Autodesk Fusion 360 part; units mm, degrees
sketch "Sketch1" plane through (0, 0, 0) normal (0, 0, 1) x (1, 0, 0)
  line L0 (0, 0) -> (18.542, 0)
  line L1 (18.542, 0) -> (18.542, 39.37)
  line L2 (18.542, 39.37) -> (0, 39.37)
  line L3 (0, 39.37) -> (0, 0)
  line L4 (3.302, 0) -> (3.302, 39.37)
  line L5 (15.24, 0) -> (15.24, 39.37)
  line L6 (16.51, 38.1) -> (17.272, 38.1)
  line L7 (17.272, 38.1) -> (17.272, 1.27)
  line L8 (17.272, 1.27) -> (16.51, 1.27)
  line L9 (16.51, 1.27) -> (16.51, 38.1)
  line L10 (1.27, 38.1) -> (2.032, 38.1)
  line L11 (2.032, 38.1) -> (2.032, 1.27)
  line L12 (2.032, 1.27) -> (1.27, 1.27)
  line L13 (1.27, 1.27) -> (1.27, 38.1)
  line L14 (-1.6611, 32.385) -> (20.0985, 32.385) construction
  line L15 (-1.6611, 6.985) -> (20.0985, 6.985) construction
  line L16 (8.9225, 41.0496) -> (8.9225, -1.9164) construction
  circle A0 centre (8.9225, 32.385) radius 2.032
  circle A1 centre (8.9225, 6.985) radius 2.032
  dimension "d1" = 18.542
  dimension "d2" = 39.37
  dimension "d3" = 3.302
  dimension "d4" = 3.302
  dimension "d5" = 36.83
  dimension "d6" = 1.27
  dimension "d7" = 0.762
  dimension "d8" = 1.27
  dimension "d9" = 36.83
  dimension "d11" = 0.762
  dimension "d12" = 1.27
  dimension "d13" = 1.27
  dimension "d26" = 6.985
  dimension "d27" = 6.985
  dimension "d28" = 4.064
  dimension "d29" = 4.064
extrude "Extrude1" add sketch "Sketch1" along normal blind 2.54 contours L0 L2 L4 L5 | A0 | A1
extrude "Extrude2" add sketch "Sketch1" along normal blind 12.7 contours L0 L1 L2 L5
extrude "Extrude3" add sketch "Sketch1" along normal blind 12.7 contours L0 L2 L3 L4
extrude "Extrude4" add sketch "Sketch1" along normal blind 6.35 contours L6 L7 L8 L9
extrude "Extrude5" add sketch "Sketch1" along normal blind 6.35 contours L10 L11 L12 L13
extrude "Extrude6" cut sketch "Sketch1" along normal through all contours A0
extrude "Extrude7" cut sketch "Sketch1" along normal through all contours A1
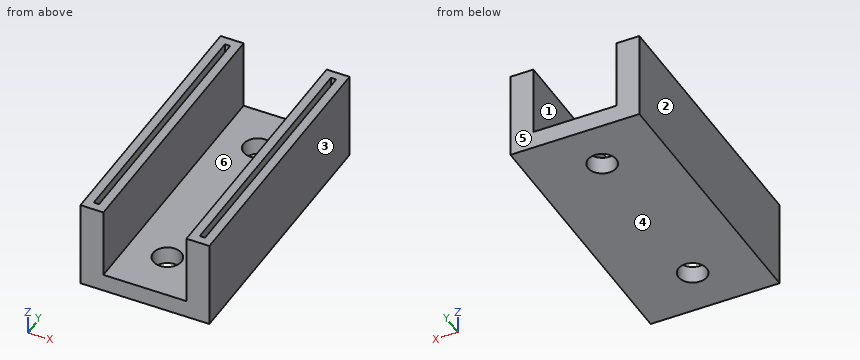
For this review, take the finished solid that the model builds, in its own axes (mm). Face numbers are marked on the shaded views. A direction names the side the tool comes from. Round coordinates to 2 decimals unless told otherwise and drop trailing zeros. Write each loop counter-clockwise with the first axis right and the second up, starting at its lowest first coordinate (ties: lowest second). Pieces come first, ordered by that corner, then holes. Notation, with made-up numbers: M -5.5,31 L 38.5,31 A16 ccw 38.5,43 Z; hole C 52,83.5 d1. An arc over 180 degrees is marked long. One line per item, written item: value. Start each with the question number.
(1) Machinability: for the marked faces 5 and 6, which of the approach directions +Z, -Z, +X, -X, +Y, -Y give a long, thin tool a straight path to every point of the face, cutting with its end or side? Answer none if there is none.
(2) We need section C-C (y = 13). Give the boundary of the cut face in (x, z), and give its area (3 significant figures).
(3) The part is to be moulded in two halves that separate along X. For the marked faces 1, 2, 3 and 4, say which applies: released by +X, released by -X, zero draft, split by the parting line, or undercut.
(4) We need section D-D (y = 34). Give the boundary of the cut face in (x, z).
(5) Wall thickness on line 1 (X direction, y = 17.5, z = 11.5); line 2 (X direction, y = 20.5, z = 4); line 3 (Z direction, x = 10.75, y = 4): over which ranges is each line inside the solid? List them lowest first.
(6) We need section B-B (z = 4). Give the boundary of the cut face in (x, y).
(7) We need section A-A (z = 7.5). Give the boundary of the cut face in (x, y), and give its area (3 significant figures).
(8) Insertion check: pin 1 (3.5 mm diameter, centred on x = 8.92, y = 6.98, fed in from -Z). The pin has a flat end and moves straight along its axis. Give the tip position at first contact, or say it passes through.
Result:
1. face 5: +Z, -Z, +X, -X, +Y
1. face 6: +Z, +Y, -Y
2. outline: M 0,0 L 18.54,0 L 18.54,12.7 L 17.27,12.7 L 17.27,6.35 L 16.51,6.35 L 16.51,12.7 L 15.24,12.7 L 15.24,2.54 L 3.3,2.54 L 3.3,12.7 L 2.03,12.7 L 2.03,6.35 L 1.27,6.35 L 1.27,12.7 L 0,12.7 Z
2. area: 105 mm²
3. face 1: undercut
3. face 2: released by -X
3. face 3: released by +X
3. face 4: zero draft
4. outline: M 0,0 L 7.69,0 L 7.69,2.54 L 3.3,2.54 L 3.3,12.7 L 2.03,12.7 L 2.03,6.35 L 1.27,6.35 L 1.27,12.7 L 0,12.7 Z; M 10.16,0 L 18.54,0 L 18.54,12.7 L 17.27,12.7 L 17.27,6.35 L 16.51,6.35 L 16.51,12.7 L 15.24,12.7 L 15.24,2.54 L 10.16,2.54 Z
5. line 1: 0 to 1.27, 2.03 to 3.3, 15.24 to 16.51, 17.27 to 18.54
5. line 2: 0 to 3.3, 15.24 to 18.54
5. line 3: 0 to 2.54
6. outline: M 0,0 L 3.3,0 L 3.3,39.37 L 0,39.37 Z; M 15.24,0 L 18.54,0 L 18.54,39.37 L 15.24,39.37 Z
7. outline: M 0,0 L 3.3,0 L 3.3,39.37 L 0,39.37 Z; M 15.24,0 L 18.54,0 L 18.54,39.37 L 15.24,39.37 Z; hole M 1.27,1.27 L 2.03,1.27 L 2.03,38.1 L 1.27,38.1 Z; hole M 16.51,1.27 L 17.27,1.27 L 17.27,38.1 L 16.51,38.1 Z
7. area: 204 mm²
8. pin 1: through
